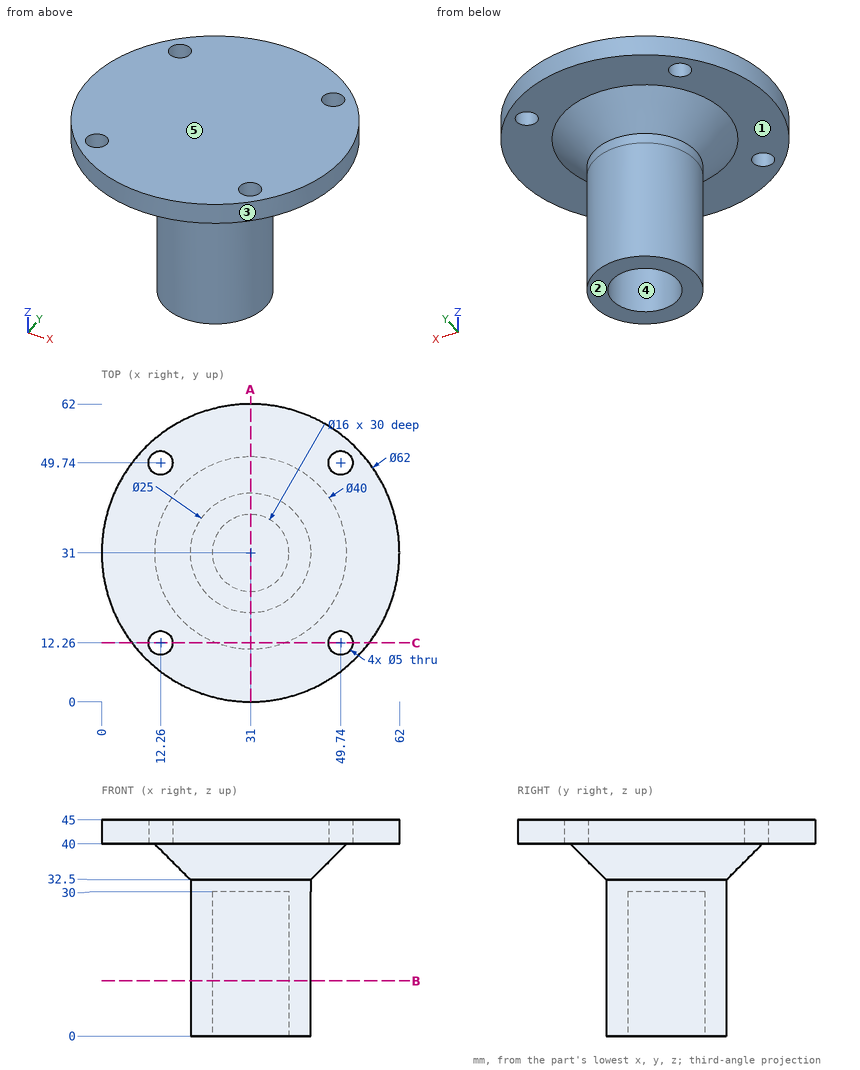
Could you check a few things on this drawing? It's one solid part, dimensions in mm from its lowest x, y, z. A direction names the side the tool comes from. Round coordinates to 2 decimals unless told otherwise and drop trailing zeros. Order: outer loops, then holes, each group sorted by start corner. A loop starts at its lowest first (then second) coordinate and runs counter-clockwise, first axis right, second up. Notation, with made-up numbers: M 69,51.25 L 114,51.25 A34 ccw 114,82.25 Z; hole C 0.25,73.25 d5. An arc over 180 degrees is marked long. One line per question, with ' | ' between items. Start each with the question number.
(1) Thinking about a two-plate mould opening in X: for the marked faces 3, 4 and 5, which applies, +X half, -X half, draft (parallel to the pull), parting line (faces both ways), or undercut?
(2) For P1, Ø10, axis at x = 46.5, z = 25, coming from the -Y side; P2, Ø6, axis at y = 45.5, z = 19.5, coming from the -X side; P3, Ø1, axis at x = 39.5, z = 17.5, coming from the -Y side, each with a flat end and sliding along its axis, tell me the tip position at first contact or that it passes through.
(3) For the marked faces 1 and 2, which set-ups out of +Z, -Z, +X, -X, +Y, -Y let a thin tool reach every point of the face, with its end or its side?
(4) Suppose I cut it at C-C on y = 12.26. Count the separate pieces of the cut face and the enclosed holes in it, then the cut area to 3 significant figures.
(5) Suppose I cut it at A-A on x = 31. List the corners of the cut face in (y, z) for me, then the cut area to 3 significant figures.
(6) Suppose I cut it at B-B on z = 11.5. List the corners of the cut face in (x, y) for me, then the cut area to 3 significant figures.
(7) Please list where these lines run through material, in increasing order: line 1 along X through (y, z) = (50, 41); line 2 along Y through (x, z) = (12.26, 41.85).
Geometry results:
1) face 3: parting line | face 4: undercut | face 5: draft
2) P1: y = 24.22 | P2: x = 26.1 | P3: y = 21.4
3) face 1: -Z | face 2: -Z, +X, -X, +Y, -Y
4) separate pieces: 3 | enclosed holes: 0 | area: 209 mm²
5) outline: M 0,40 L 11,40 L 18.5,32.5 L 18.5,0 L 23,0 L 23,30 L 39,30 L 39,0 L 43.5,0 L 43.5,32.5 L 51,40 L 62,40 L 62,45 L 0,45 Z | area: 886 mm²
6) outline: C 31,31 d25; hole C 31,31 d16 | area: 290 mm²
7) line 1: 6.51 to 9.77, 14.75 to 47.25, 52.23 to 55.49 | line 2: 6.31 to 9.76, 14.76 to 47.24, 52.24 to 55.69
